Could you check a few things on this model? Use its own coordinates, in mm. Give positions to 0.01 mm unless a question says otherwise; leave off trailing zeros. Order: outer loops, then holes, each group sorted by start corner. A loop starts at its lowest first (then second) coordinate and runs counter-clockwise, first axis right, second up. Notation, with made-up numbers: (-22, 89.25) -> (-6, 89.25) arc R36 ccw to (-6, 126.25) -> close; hole circle Ø1 at (58, -12.5). An arc over 180 degrees is marked (long way). Write each question's results on one line, items separated by ' | '.
```python
from build123d import *

# Parameters (mm, degrees)
SALIENTE_EXTRUIR1_DEPTH = 5
CROQUIS2_W              = 26.666666666
CROQUIS2_H              = 5
CORTAR_EXTRUIR1_DEPTH   = 10
CORTAR_EXTRUIR3_DEPTH   = 10


with BuildPart() as part:
    # Croquis1 → Saliente-Extruir1 (new body)
    with BuildSketch(Plane.XY):
        Polygon((0, 28.333333333), (0, 5), (26.666666667, 5), (26.666666667, 0), (53.333333333, 0), (53.333333333, 5), (80, 5), (80, 28.333333333), (75, 28.333333333), (75, 51.666666667), (80, 51.666666667), (80, 75), (0, 75), (0, 51.666666667), (5, 51.666666667), (5, 28.333333333), align=None)
    extrude(amount=SALIENTE_EXTRUIR1_DEPTH)

    # Croquis2 → Cortar-Extruir1 (cut)
    with BuildSketch(Plane.XY.offset(5)):
        with Locations((40, 72.5)):
            Rectangle(CROQUIS2_W, CROQUIS2_H)
    extrude(amount=-CORTAR_EXTRUIR1_DEPTH, mode=Mode.SUBTRACT)

    # Croquis5 → Cortar-Extruir3 (cut)
    with BuildSketch(Plane.XY.offset(5)):
        with BuildLine():
            ThreePointArc((46, 40), (44.242640687, 44.242640687), (40, 46))
            Line((40, 46), (40, 40))
            Line((40, 40), (46, 40))
        make_face()
        with BuildLine():
            Line((40, 40), (40, 46))
            ThreePointArc((40, 46), (35.757359313, 35.757359313), (46, 40))
            Line((46, 40), (40, 40))
        make_face()
    extrude(amount=-CORTAR_EXTRUIR3_DEPTH, mode=Mode.SUBTRACT)


solid = part.part
```
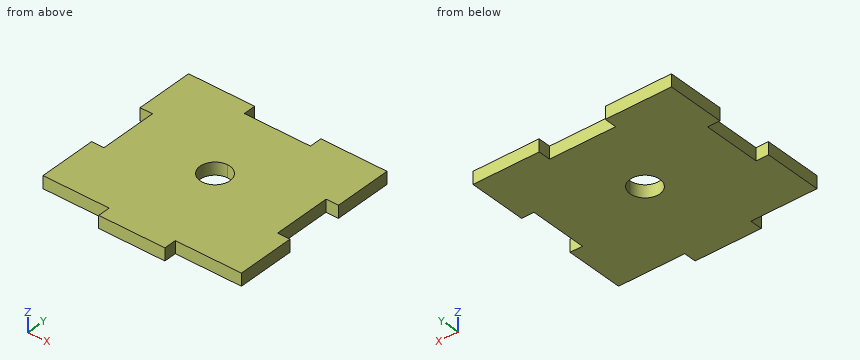
Q1. Suppose I cut it at B-B on y = 36. Please give me the cut outline in (x, z).
Here are the results:
outline: (5, 0) -> (35.53, 0) -> (35.53, 5) -> (5, 5) -> close; (44.47, 0) -> (75, 0) -> (75, 5) -> (44.47, 5) -> close
Q2. Suppose I cut it at A-A on z = 2.3. Please give me the cut outline in (x, y).
Here are the results:
outline: (0, 5) -> (26.67, 5) -> (26.67, 0) -> (53.33, 0) -> (53.33, 5) -> (80, 5) -> (80, 28.33) -> (75, 28.33) -> (75, 51.67) -> (80, 51.67) -> (80, 75) -> (53.33, 75) -> (53.33, 70) -> (26.67, 70) -> (26.67, 75) -> (0, 75) -> (0, 51.67) -> (5, 51.67) -> (5, 28.33) -> (0, 28.33) -> close; hole circle Ø12 at (40, 40)
Q3. Suppose I cut it at C-C on x = 7.5. Please give me the cut outline in (y, z), and give its area (3 significant figures).
Here are the results:
outline: (5, 0) -> (75, 0) -> (75, 5) -> (5, 5) -> close | area: 350 mm²
Q4. I'm going to push flat-ended pins straight in: pin 1 Ø1.5 at (y, z) = (39.5, 2) entering from +X; pin 2 Ø1.5 at (y, z) = (35.5, 3.5) entering from -X; pin 3 Ø3 at (x, z) = (29, 3) entering from +Y. Where does each tip first touch, or does it pass through?
Here are the results:
pin 1: stops at x = 75 | pin 2: stops at x = 5 | pin 3: stops at y = 70
Q5. I need wall thicknesses on line 1 along Y through (x, z) = (40, 3.05); line 2 along X through (y, z) = (40, 1); line 3 along Y through (x, z) = (19, 1.05). Which ranges of each line are inside material? Lowest first, please.
Here are the results:
line 1: y = 0 to 34, 46 to 70 | line 2: x = 5 to 34, 46 to 75 | line 3: y = 5 to 75
